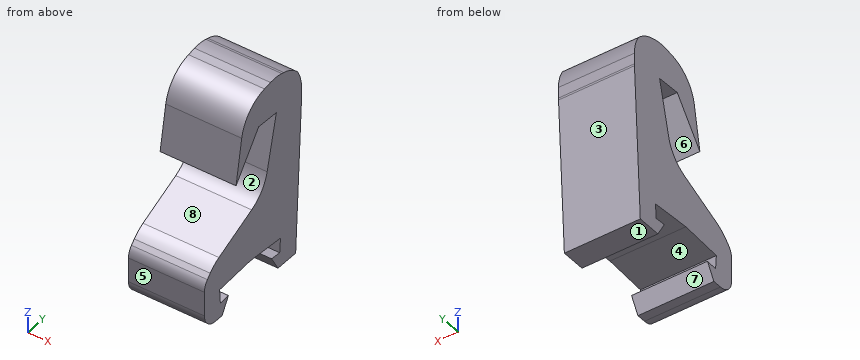
from build123d import *

# Parameters (mm, degrees)
F2_DEPTH     = 10
F3_T1_DEPTH  = 10
F3_T3_DEPTH  = 10.6551499426
F3_T5_DEPTH  = 18.2363272352
F3_T7_DEPTH  = 18.9745597366
F3_T9_DEPTH  = 15.1812109951
F3_T11_DEPTH = 27.7044164166
F3_T13_DEPTH = 14.9256552594
F4_R         = 2


# Not quite as in the source:
# - a fillet or chamfer that OpenCascade refuses, or shapes differently, is made with other operations: its cross-section is extruded or revolved along the edge and cut away or added


with BuildPart() as f2:
    # F1 (on Right) → F2 (new body)
    with BuildSketch(Plane.YZ):
        Polygon((-5.0547005384, 0), (-3.9, 2), (-5.3636236598, 1.894673786), (-5.5, 3.7897731222), (0, 4.18556761), (5.5, 3.7897731222), (5.3636236598, 1.894673786), (3.9, 2), (5.0547005384, 0), (8.2396483049, 0), (9.3, 20.2171942833), (9.3, 23.4340857714), (7.8309578478, 25.4216119647), (4.720045685, 26.1993408203), (-0.8888025768, 25.2726981416), (-2.5269729085, 15.9901147708), (1.5650866553, 21.3901147708), (4.7629482978, 21.2731493252), (2.5189220905, 11.9409952313), (-6.5113636665, 7.8363195062), (-8.2396483049, 6), (-8.2396483049, 0), align=None)
    extrude(amount=F2_DEPTH)

    # F3: fillet of radius 5 on 7 edges, made by hand

    # F3_s2 → F3_t1 (join)
    with BuildSketch(Plane.YZ):
        with BuildLine():
            ThreePointArc((3.0895210417, 14.313925334), (2.0840852214, 12.299936757), (0.2971092897, 10.9310802281))
            Line((0.2971092897, 10.9310802281), (2.5189220905, 11.9409952313))
            Line((2.5189220905, 11.9409952313), (3.0895210417, 14.313925334))
        make_face()
    extrude(amount=F3_T1_DEPTH)

    # F3_s4 → F3_t3 (cut)
    with BuildSketch(Plane.YZ.offset(-0.3275749713)):
        with BuildLine():
            ThreePointArc((9.2931371699, 20.0863441421), (9.298283998, 20.2172392528), (9.3, 20.3482242718))
            Line((9.3, 20.3482242718), (9.3, 20.2171942833))
            Line((9.3, 20.2171942833), (9.2931371699, 20.0863441421))
        make_face()
    extrude(amount=F3_T3_DEPTH, mode=Mode.SUBTRACT)

    # F3_s6 → F3_t5 (cut)
    with BuildSketch(Plane.YZ.offset(-4.1181636176)):
        with BuildLine():
            ThreePointArc((9.3, 21.7868203244), (9.0489155839, 23.3513652349), (8.3208796893, 24.7587770072))
            Line((8.3208796893, 24.7587770072), (9.3, 23.4340857714))
            Line((9.3, 23.4340857714), (9.3, 21.7868203244))
        make_face()
    extrude(amount=F3_T5_DEPTH, mode=Mode.SUBTRACT)

    # F3_s8 → F3_t7 (cut)
    with BuildSketch(Plane.YZ.offset(-4.4872798683)):
        with BuildLine():
            ThreePointArc((6.089637591, 25.856942485), (7.6572398301, 25.1619533788), (8.8978379592, 23.9781869661))
            Line((8.8978379592, 23.9781869661), (7.8309578478, 25.4216119647))
            Line((7.8309578478, 25.4216119647), (6.089637591, 25.856942485))
        make_face()
    extrude(amount=F3_T7_DEPTH, mode=Mode.SUBTRACT)

    # F3_s10 → F3_t9 (cut)
    with BuildSketch(Plane.YZ.offset(-2.5906054975)):
        with BuildLine():
            ThreePointArc((3.6976623422, 26.0304319828), (4.715730589, 26.0931776147), (5.7253482208, 25.948014923))
            Line((5.7253482208, 25.948014923), (4.720045685, 26.1993408203))
            Line((4.720045685, 26.1993408203), (3.6976623422, 26.0304319828))
        make_face()
    extrude(amount=F3_T9_DEPTH, mode=Mode.SUBTRACT)

    # F3_s12 → F3_t11 (cut)
    with BuildSketch(Plane.YZ.offset(-8.8522082083)):
        with BuildLine():
            ThreePointArc((-1.5041807088, 21.7856988327), (-0.0963977073, 24.4715707073), (2.6047244105, 25.8498667607))
            Line((2.6047244105, 25.8498667607), (-0.8888025768, 25.2726981416))
            Line((-0.8888025768, 25.2726981416), (-1.5041807088, 21.7856988327))
        make_face()
    extrude(amount=F3_T11_DEPTH, mode=Mode.SUBTRACT)

    # F3_s14 → F3_t13 (cut)
    with BuildSketch(Plane.YZ.offset(-2.4628276297)):
        with BuildLine():
            ThreePointArc((-5.6145333952, 8.2439696673), (-6.4554211776, 7.7581509396), (-7.1865343837, 7.1189439476))
            Line((-7.1865343837, 7.1189439476), (-6.5113636665, 7.8363195062))
            Line((-6.5113636665, 7.8363195062), (-5.6145333952, 8.2439696673))
        make_face()
    extrude(amount=F3_T13_DEPTH, mode=Mode.SUBTRACT)

    # F4
    f4_edges = [f2.edges().sort_by_distance(p)[0] for p in [
        (5, -8.239648, 0),
        (5, -8.239648, 6),
    ]]
    fillet(f4_edges, radius=F4_R)


solid = f2.part
The listing builds one solid part. Answer for the finished solid, in the listing's coordinates (mm). Face numbers are marked on the shaded views. A direction names the side the tool comes from. Coordinates: 2 decimals unless noted, no trailing zeros. Loops run counter-clockwise (first coordinate to the right, second up) from the corner with the lowest first, then second, coordinate; pieces in that order, holes last. Notation, with made-up numbers: M 2,-17.75 L 16,-17.75 A17 cw 16,13.25 Z; hole C 39.25,18.5 d5. An arc over 180 degrees is marked long. Answer in a Markdown table with one row per item.
1) Which of the six approach directions +Z, -Z, +X, -X, +Y, -Y give full straight-line access (tool end or side, diameter ignored) to the marked faces 5, 6, 7 and 8?
Answers below:
| item | result |
|---|---|
| face 5 | +Z, -Z, +X, -X, -Y |
| face 6 | +X, -X |
| face 7 | -Z, +X, -X |
| face 8 | +X, -X, -Y |
2) Determine the mould class of the marked faces 1, 2, 3 and 4 for opening direction Y: released by +Y, released by -Y, zero draft, split by the parting line, or undercut.
Answers below:
| item | result |
|---|---|
| face 1 | zero draft |
| face 2 | released by -Y |
| face 3 | released by +Y |
| face 4 | undercut |
3) Given pin 1 (5 mm diameter, centred on x = 6.5, y = 1.5, fed in from +Z); pin 2 (5 mm diameter, centred on x = 4.5, z = 16.5, fed in from +Y); pin 3 (2 mm diameter, centred on x = 5.5, z = 13, fed in from -Y), each flat-ended and moving along its own axis, determine where each tip first touches the part or whether it passes through.
Answers below:
| item | result |
|---|---|
| pin 1 | z = 26.07 |
| pin 2 | y = 9.24 |
| pin 3 | y = 1.82 |
4) Find section A-A (z = 2.75). Determine the outline of the cut face in (x, y), then the cut area to 3 significant figures.
Answers below:
| item | result |
|---|---|
| outline | M 0,-8.24 L 10,-8.24 L 10,-5.43 L 0,-5.43 Z; M 0,5.43 L 10,5.43 L 10,8.38 L 0,8.38 Z |
| area | 57.7 mm^2 |
5) Find section D-D (y = 7). Determine the outline of the cut face in (x, z), then the cut area to 3 significant figures.
Answers below:
| item | result |
|---|---|
| outline | M 0,0 L 10,0 L 10,25.53 L 0,25.53 Z |
| area | 255 mm^2 |
6) Find section C-C (y = 2.25). Determine the outline of the cut face in (x, z).
Answers below:
| item | result |
|---|---|
| outline | M 0,4.02 L 10,4.02 L 10,12.51 L 0,12.51 Z; M 0,21.37 L 10,21.37 L 10,25.78 L 0,25.78 Z |
7) Find the intervals of material crossed by probe 1 along Z at (x, y) = (7.75, -4.5); probe 2 along Y at (x, z) = (7, 18.75); probe 3 along Y at (x, z) = (4, 2.5), in increasing order.
Answers below:
| item | result |
|---|---|
| probe 1 | 0.96 to 1.96, 3.86 to 8.75 |
| probe 2 | -2.04 to -0.44, 4.16 to 9.22 |
| probe 3 | -8.24 to -5.41, 5.41 to 8.37 |
